CAD build for the part. Positions are in the model's coordinates, mm. Give positions to 0.01 mm unless a question says otherwise; leave off trailing zeros. Order: outer loops, then holes, each group sorted by start corner. A loop starts at its lowest first (then second) coordinate and runs counter-clockwise, first axis right, second up. Notation, with made-up numbers: (6.25, -6.75) -> (12.25, -6.75) arc R14 ccw to (12.25, -1.75) -> close; hole circle Ø2 at (-27, 72). An arc over 180 degrees is marked (long way). Use one line per item in the form item = value. Start each with the question number.
1) Cut at D-D, the plane z = -46. Give the cut face in (x, y).
2) Drop flat-ended pins along their axis: P1, Ø16, axis at x = -659.5, y = -13, coming from the -Z side; P2, Ø2, axis at x = 72.5, y = 15.5, coming from the -Z side; P3, Ø12, axis at y = 17.5, z = -99, coming from the +X side. Give the stop position or say it passes through.
3) Cut at A-A, the plane x = -171. Give the cut face in (y, z).
4) Probe line 1 (Y direction, x = -804, z = -25.5); line 2 (Z direction, x = -256, y = -15); line 3 (X direction, y = -22, z = -48). List the from-to ranges inside material, lowest first.
5) Cut at B-B, the plane y = 15.5. Give the cut face in (x, z).
6) Cut at C-C, the plane z = 0. Give the cut face in (x, y), and give its area (3 significant figures).
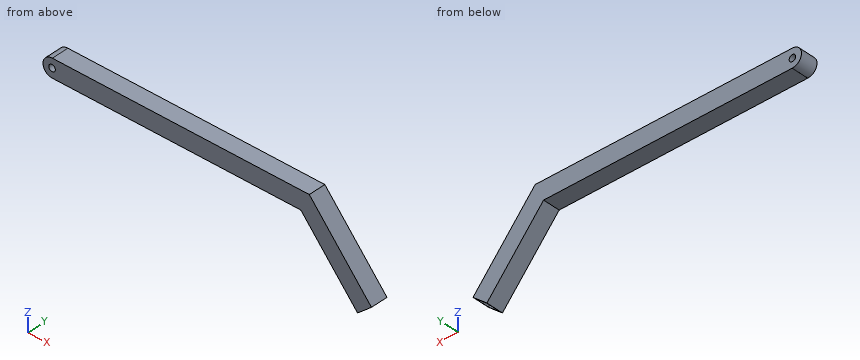
from build123d import *

# Parameters (mm, degrees)
F2_W          = 62.2634254396
F2_H          = 66.4744749665
F2_W_2        = 53.8413152099
F2_H_2        = 57.4507899582
F4_R          = 33.0786713832
F5_DEPTH      = 31.1317127198
F5_DEPTH_BACK = 31.1317127198
F6_R          = 11.9370670554
F7_DEPTH      = 62.2634254396


with BuildPart() as f3:
    # F3: sweep along a path in F0
    with BuildLine(Plane.XZ) as f3_path:
        Line((-920.0506210327, 0), (0, 0))
        Line((0, 0), (216.415554285, -253.3791065216))
    # F2 (on plane+point) → F3 (sweep)
    with BuildSketch(Plane.YZ.offset(-920.0506210327)):
        Rectangle(F2_W, F2_H)
        Rectangle(F2_W_2, F2_H_2, mode=Mode.SUBTRACT)
    sweep(path=f3_path.line, transition=Transition.RIGHT)

    # F4 (on Front) → F5 (join, two sides)
    with BuildSketch(Plane.XZ) as f5_sk:
        with Locations((-920.9526777267, 0)):
            Circle(F4_R)
    extrude(amount=F5_DEPTH)
    extrude(f5_sk.sketch, amount=-F5_DEPTH_BACK)

    # F6 (on face) → F7 (cut, through all)
    with BuildSketch(Plane(origin=(0, 31.1317127198, 0), x_dir=(-1, 0, 0), z_dir=(0, 1, 0))):
        with Locations((920.9526777267, 0)):
            Circle(F6_R)
    extrude(amount=-F7_DEPTH, mode=Mode.SUBTRACT)


solid = f3.part
Result:
q1.outline = (-4.42, -31.13) -> (83, -31.13) -> (83, 31.13) -> (-4.42, 31.13) -> close; hole (1.51, -26.92) -> (77.07, -26.92) -> (77.07, 26.92) -> (1.51, 26.92) -> close
q2.P1 = -33.24
q2.P2 = -137.23
q2.P3 = 133.39
q3.outline = (-31.13, -33.24) -> (31.13, -33.24) -> (31.13, 33.24) -> (-31.13, 33.24) -> close; hole (-26.92, -28.73) -> (26.92, -28.73) -> (26.92, 28.73) -> (-26.92, 28.73) -> close
q4.line_1 = -31.13 to -26.92, 26.92 to 31.13
q4.line_2 = -33.24 to -28.73, 28.73 to 33.24
q4.line_3 = -2.71 to 3.22, 78.77 to 84.71
q5.outline = (-920.05, -33.24) -> (-15.32, -33.24) -> (191.14, -274.97) -> (194.57, -272.04) -> (-13.24, -28.73) -> (-904.55, -28.73) arc R33.08 ccw to (-904.55, 28.73) -> (13.24, 28.73) -> (238.26, -234.72) -> (241.69, -231.79) -> (15.32, 33.24) -> (-920.05, 33.24) -> (-920.05, 33.07) arc R33.08 ccw (long way) to (-920.05, -33.07) -> close; hole circle Ø23.87 at (-920.95, 0)
q6.outline = (-954.03, -31.13) -> (-932.89, -31.13) -> (-932.89, 31.13) -> (-954.03, 31.13) -> close; (-909.02, -31.13) -> (43.71, -31.13) -> (43.71, 31.13) -> (-909.02, 31.13) -> close; hole (-887.87, -26.92) -> (37.78, -26.92) -> (37.78, 26.92) -> (-887.87, 26.92) -> close
q6.area = 10,800 mm²
